Here's how the part is built. I have some questions about the finished solid (model axes, mm). Face numbers are marked on the shaded views. A direction names the side the tool comes from. Coordinates: 2 decimals unless noted, no trailing zeros. Write each loop counter-clockwise with the first axis right and the second up, starting at its lowest first coordinate (ties: lowest second). Pieces come first, ordered by that corner, then holes.
Item 1: I want a section at A-A (y = 0). Please give me the cut outline in (x, z), and give its area (3 significant figures).
Item 2: I want a section at C-C (y = -9.25). Please give me the cut outline in (x, z).
Item 3: I want a section at B-B (z = 0). Please give me the cut outline in (x, y), and give its area (3 significant figures).
Item 4: For the marked faces 1 and 2, which set-ups out of +Z, -Z, +X, -X, +Y, -Y let a thin tool reach every point of the face, with its end or its side?
Item 5: I want a section at D-D (x = 34). Please give me the cut outline in (y, z), and give its area (3 significant figures).
Item 6: I'm going to push flat-ended pins straight in: P1, Ø16.5, axis at y = 7.5, z = 0, coming from the +X side; P2, Ø1.5, axis at y = 7.5, z = 4, coming from the +X side; P3, Ø16, axis at x = 30.04, y = 0, coming from the +Z side; P4, Ø10, axis at y = -6.5, z = -4, coming from the -X side. Where does each tip first touch, or does it pass through?
Item 7: Please list where these lines run through material, in increasing order: line 1 (Z direction, x = -40, y = 10.25); line 2 (X direction, y = 11.5, z = 3.75); line 3 (X direction, y = 5.25, z = 9).
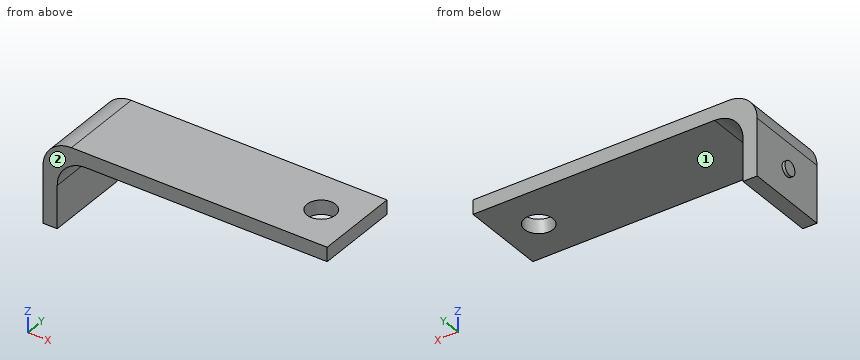
from build123d import *

# Parameters (mm, degrees)
BOSS_EXTRUDE1_DEPTH = 15
SKETCH2_R           = 5
CUT_EXTRUDE1_DEPTH  = 30
SKETCH3_R           = 2.5
BOSS_EXTRUDE2_DEPTH = 1


with BuildPart() as part:
    # Sketch1 → Boss-Extrude1 (new, symmetric)
    with BuildSketch(Plane(origin=(0, 0, 0), x_dir=(1, 0, 0), z_dir=(0, 1, 0))):
        with BuildLine():
            Line((-57.34741784, 10.399061033), (-52.34741784, 10.399061033))
            Line((-52.34741784, 10.399061033), (-52.34741784, -4.600938967))
            ThreePointArc((-52.34741784, -4.600938967), (-49.418485652, -11.672006779), (-42.34741784, -14.600938967))
            Line((-42.34741784, -14.600938967), (42.65258216, -14.600938967))
            Line((42.65258216, -14.600938967), (42.65258216, -19.600938967))
            Line((42.65258216, -19.600938967), (-47.34741784, -19.600938967))
            ThreePointArc((-47.34741784, -19.600938967), (-54.418485652, -16.672006779), (-57.34741784, -9.600938967))
            Line((-57.34741784, -9.600938967), (-57.34741784, 10.399061033))
        make_face()
    extrude(amount=BOSS_EXTRUDE1_DEPTH, both=True)

    # Sketch2 → Cut-Extrude1 (cut)
    with BuildSketch(Plane(origin=(0, 0, 14.600938967), x_dir=(-1, 0, 0), z_dir=(0, 0, -1))):
        with Locations((-30.040799479, 0)):
            Circle(SKETCH2_R)
    extrude(amount=-CUT_EXTRUDE1_DEPTH, mode=Mode.SUBTRACT)

    # Sketch3 → Boss-Extrude2 (add)
    with BuildSketch(Plane.ZY.offset(57.34741784)):
        with Locations(Location((0, 0, 0), (0, 0, 180))):
            Circle(SKETCH3_R)
    extrude(amount=BOSS_EXTRUDE2_DEPTH)


solid = part.part
Answer:
1. outline: (-58.35, -2.5) - (-57.35, -2.5) - (-57.35, -10.4) - (-52.35, -10.4) - (-52.35, 4.6) arc R10 cw to (-42.35, 14.6) - (25.04, 14.6) - (25.04, 19.6) - (-47.35, 19.6) arc R10 ccw to (-57.35, 9.6) - (-57.35, 2.5) - (-58.35, 2.5) - close; (35.04, 14.6) - (42.65, 14.6) - (42.65, 19.6) - (35.04, 19.6) - close
1. area: 580 mm2
2. outline: (-57.35, -10.4) - (-52.35, -10.4) - (-52.35, 4.6) arc R10 cw to (-42.35, 14.6) - (42.65, 14.6) - (42.65, 19.6) - (-47.35, 19.6) arc R10 ccw to (-57.35, 9.6) - close
3. outline: (-58.35, -2.5) - (-57.35, -2.5) - (-57.35, -15) - (-52.35, -15) - (-52.35, 15) - (-57.35, 15) - (-57.35, 2.5) - (-58.35, 2.5) - close
3. area: 155 mm2
4. face 1: -Z, +X, +Y, -Y
4. face 2: +Z, -Z, +X, -X, -Y
5. outline: (-15, 14.6) - (-3.05, 14.6) - (-3.05, 19.6) - (-15, 19.6) - close; (3.05, 14.6) - (15, 14.6) - (15, 19.6) - (3.05, 19.6) - close
5. area: 119 mm2
6. P1: stops at x = -51.66
6. P2: stops at x = -52.35
6. P3: stops at z = 19.6
6. P4: stops at x = -57.35
7. line 1: z = 14.6 to 19.6
7. line 2: x = -57.35 to -52.35
7. line 3: x = -57.35 to -51.33
